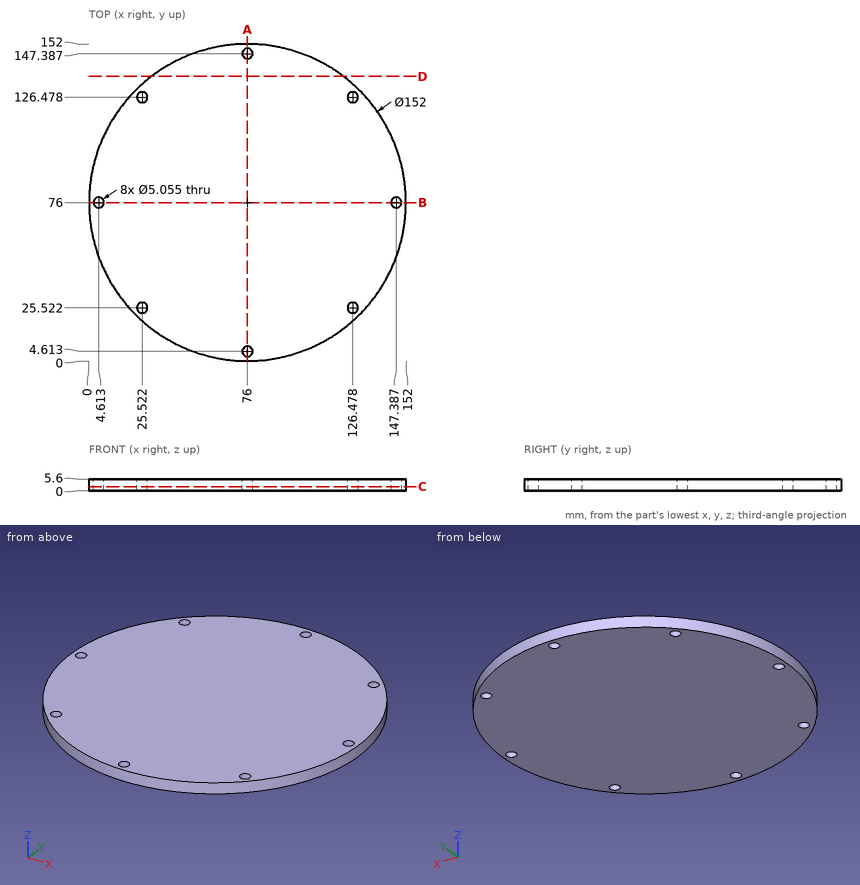
Drawing for the job (mm, zero at the part's lowest x, y, z). Round coordinates to 2 decimals unless told otherwise and drop trailing zeros. Write each loop counter-clockwise with the first axis right and the second up, starting at its lowest first coordinate (ties: lowest second). Pieces come first, ordered by that corner, then holes. Notation, with made-up numbers: M 46.5,74.25 L 58.5,74.25 A10 ccw 58.5,88.25 Z; hole C -36,75 d1. An arc over 180 degrees is marked long. Answer as a JSON object with one key per item and string values. Group by question number.
(1) Cut at D-D (y = 136.5). Give the cut face in (x, z).
(2) Flat gauge pin, fed straight in: pin 1 (1 mm diameter, centred on x = 135.5, z = 5, fed in from -Y) (1 decimal). Where does the tip first touch, or does it go through?
(3) Cut at A-A (x = 76). Give the cut face in (y, z).
(4) Cut at C-C (z = 1.9). Give the number of separate pieces and of enclosed holes in the cut face, and give its area (3 significant figures).
(5) Drill centre lines: L1, parallel to Y at x = 76, z = 2.9; L2, parallel to Y at x = 26.5, z = 0.7; L3, parallel to Y at x = 132.5, z = 1.4. Where is each one in solid material? Low to high.
Responses:
{
 "1": {"outline": "M 30,0 L 122,0 L 122,5.6 L 30,5.6 Z"},
 "2": {"pin 1": "stops at y = 28.1"},
 "3": {"outline": "M 0,0 L 2.09,0 L 2.09,5.6 L 0,5.6 Z; M 7.14,0 L 144.86,0 L 144.86,5.6 L 7.14,5.6 Z; M 149.91,0 L 152,0 L 152,5.6 L 149.91,5.6 Z"},
 "4": {"separate pieces": "1", "enclosed holes": "8", "area": "18,000 mm2"},
 "5": {"L1": "y = 0 to 2.09, 7.14 to 144.86, 149.91 to 152", "L2": "y = 18.33 to 23.19, 27.85 to 124.15, 128.81 to 133.67", "L3": "y = 25.17 to 126.83"}
}
